from build123d import *

# Parameters (mm, degrees)
BOSS_EXTRUDE1_DEPTH = 22
SKETCH3_R           = 1.75
CUT_EXTRUDE1_DEPTH  = 22
SKETCH4_R           = 3.25
CUT_EXTRUDE2_DEPTH  = 22
SKETCH5_W           = 35.231138993
SKETCH5_H           = 1
CUT_EXTRUDE3_DEPTH  = 22


with BuildPart() as part:
    # Sketch2 → Boss-Extrude1 (new body)
    with BuildSketch(Plane(origin=(0, 0, 0), x_dir=(1, 0, 0), z_dir=(0, 1, 0))):
        with BuildLine():
            Line((4.898979486, -1), (17.47140521, -1))
            ThreePointArc((17.47140521, -1), (0, -17.5), (-17.47140521, -1))
            Line((-17.47140521, -1), (-4.898979486, -1))
            ThreePointArc((-4.898979486, -1), (0, -5), (4.898979486, -1))
        make_face()
    extrude(amount=BOSS_EXTRUDE1_DEPTH)

    # Sketch3 → Cut-Extrude1 (cut)
    with BuildSketch(Plane(origin=(0, 0, 1), x_dir=(-1, 0, 0), z_dir=(0, 0, -1))):
        with Locations((11.185192348, 11)):
            Circle(SKETCH3_R)
        with Locations((-11.185192348, 11)):
            Circle(SKETCH3_R)
    extrude(amount=-CUT_EXTRUDE1_DEPTH, mode=Mode.SUBTRACT)

    # Sketch4 → Cut-Extrude2 (cut)
    with BuildSketch(Plane(origin=(0, 0, 5), x_dir=(-1, 0, 0), z_dir=(0, 0, -1))):
        with Locations((-11.185192348, 11)):
            Circle(SKETCH4_R)
        with Locations((11.185192348, 11)):
            Circle(SKETCH4_R)
    extrude(amount=-CUT_EXTRUDE2_DEPTH, mode=Mode.SUBTRACT)

    # Sketch5 → Cut-Extrude3 (cut)
    with BuildSketch(Plane(origin=(0, 22, 0), x_dir=(1, 0, 0), z_dir=(0, 1, 0))):
        with Locations((0.144164287, -1.5)):
            Rectangle(SKETCH5_W, SKETCH5_H)
    extrude(amount=-CUT_EXTRUDE3_DEPTH, mode=Mode.SUBTRACT)


solid = part.part
Work out the finished part from the listing and answer in its coordinate system (mm). A direction names the side the tool comes from. Round coordinates to 2 decimals unless told otherwise and drop trailing zeros. Loops run counter-clockwise (first coordinate to the right, second up) from the corner with the lowest first, then second, coordinate; pieces in that order, holes last. Notation, with made-up numbers: (20.5, 28) - (25.5, 28) arc R25 ccw to (25.5, 44) - close; hole circle Ø4 at (38.25, 62). An arc over 180 degrees is marked (long way). Use one line per item in the form item = value. Start each with the question number.
(1) Flat-ended cylindrical pins translate along their axes: P1, Ø1.5, axis at y = 11.5, z = 14, coming from the -X side; P2, Ø3, axis at x = -10, y = 11.5, coming from the +Z side; P3, Ø3, axis at x = 11.19, y = 11, coming from the -Z side; P4, Ø5, axis at x = 5, y = 14.5, coming from the +Z side. Find the tip coordinate at first contact, or state that the pin passes through.
(2) Find section C-C on z = 8.5. Determine the outline of the cut face in (x, y).
(3) Find section D-D on y = 13.25. Determine the outline of the cut face in (x, z).
(4) Find section B-B on x = 9. Determine the outline of the cut face in (y, z).
(5) Which of the six approach directions +Z, -Z, +X, -X, +Y, -Y give full straight-line access (tool end or side, diameter ignored) to faces 4 (the face through (0, 11, 5)), 5 (the face through (-7.94, 11.14, 9.05))?
(6) Find section A-A on y = 10. Determine the outline of the cut face in (x, z), and give its area (3 significant figures).
(7) Consider line 1 (Y direction, x = -11, z = 8.5); line 2 (X direction, y = 13, z = 10); line 3 (X direction, y = 11, z = 7.5). Determine where each line is inside the solid, lowest interval first.
(8) Determine the mould class of faces 1 (the face through (8.18, 9.76, 9.05)), 2 (the face through (0, 0, 10)), 3 (the face through (0.357, 10.846, 17.496)) for opening direction X: +X half, -X half, draft (parallel to the pull), parting line (faces both ways), or undercut.
Answer list:
q1.P1 = -8.19
q1.P2 = 5
q1.P3 = through
q1.P4 = 17.32
q2.outline = (-15.3, 0) - (15.3, 0) - (15.3, 22) - (-15.3, 22) - close; hole circle Ø6.5 at (-11.19, 11); hole circle Ø6.5 at (11.19, 11)
q3.outline = (-17.39, 2) - (-4.58, 2) arc R5 cw to (4.58, 2) - (17.39, 2) arc R17.5 ccw to (13.53, 11.1) - (13.53, 5) - (8.84, 5) - (8.84, 15.1) arc R17.5 ccw to (-8.84, 15.1) - (-8.84, 5) - (-13.53, 5) - (-13.53, 11.1) arc R17.5 ccw to start
q4.outline = (0, 2) - (22, 2) - (22, 15.01) - (13.41, 15.01) - (13.41, 5) - (8.59, 5) - (8.59, 15.01) - (0, 15.01) - close
q5.face_4 = -Z, +Y, -Y
q5.face_5 = +Z
q6.outline = (-17.39, 2) - (-12.62, 2) - (-12.62, 5) - (-14.28, 5) - (-14.28, 10.12) arc R17.5 ccw to start; (-9.75, 2) - (-4.58, 2) arc R5 cw to (4.58, 2) - (9.75, 2) - (9.75, 5) - (8.09, 5) - (8.09, 15.52) arc R17.5 ccw to (-8.09, 15.52) - (-8.09, 5) - (-9.75, 5) - close; (12.62, 2) - (17.39, 2) arc R17.5 ccw to (14.28, 10.12) - (14.28, 5) - (12.62, 5) - close
q6.area = 272 mm^2
q7.line_1 = 0 to 7.76, 14.24 to 22
q7.line_2 = -14.36 to -13.75, -8.62 to 8.62, 13.75 to 14.36
q7.line_3 = -15.81 to -14.44, -7.94 to 7.94, 14.44 to 15.81
q8.face_1 = undercut
q8.face_2 = draft
q8.face_3 = parting line
